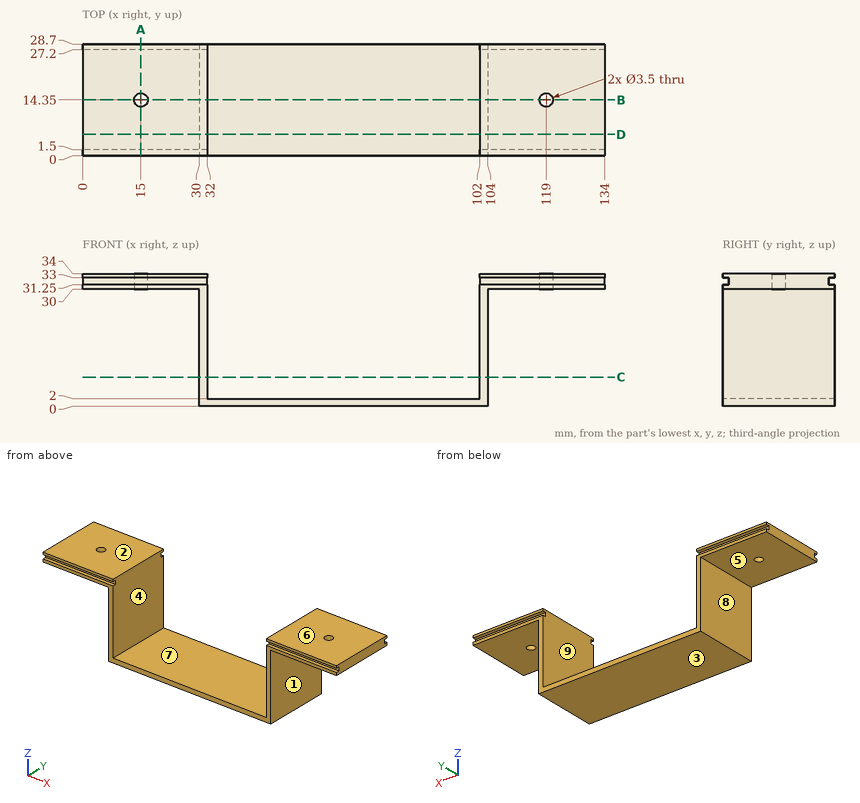
Can you work these out from the drawing? Everything is in mm from the part's minimum corner. A direction names the side the tool comes from. Coordinates: 2 decimals unless noted, no trailing zeros. Loops run counter-clockwise (first coordinate to the right, second up) from the corner with the lowest first, then second, coordinate; pieces in that order, holes last.
1) Which directions (+Z, -Z, +X, -X, +Y, -Y) give clear straight access to the entire face, cutting with the end or side of a thin tool? Please do the marked faces 1, 2, 3, 4 and 5.
2) Imagine slicing it at A-A on x = 15. List the corners of the cut face in (y, z) for me.
3) For pin 1 (1.4 mm diameter, centred on x = 112.5, z = 32, fed in from +Y); pin 2 (1 mm diameter, centred on x = 63, z = 4, fed in from +Y); pin 3 (0.5 mm diameter, centred on x = 115, z = 32.5, fed in from -Y); pin 4 (2 mm diameter, centred on x = 95, y = 13, fed in from +Z), each with a flat end and sliding along its axis, tell me the tip position at first contact or that it passes through.
4) Imagine slicing it at C-C on z = 7.5. List the corners of the cut face in (x, y) for me.
5) Thinking about a two-plate mould opening in X: for the marked faces 6, 7, 8 and 9, which applies, pulls with the +X half, pulls with the -X half, needs draft (parallel to the pull), parting line crosses it, or undercut?
6) I need wall thicknesses on probe 1 along X at (y, z) = (14.35, 32.35); probe 2 along X at (y, z) = (13.5, 30.5); probe 3 along Y at (x, z) = (15, 32.15). Which ranges of each line are inside material? Lowest first, please.
7) Imagine slicing it at D-D on y = 5.5. List the corners of the cut face in (x, z) for me, plus the area to 3 significant figures.
8) Imagine slicing it at B-B on y = 14.35. List the corners of the cut face in (x, z) for me, plus the area to 3 significant figures.
Completed:
1. face 1: -Z, +X, +Y, -Y
1. face 2: +Z, +X, -X, +Y, -Y
1. face 3: -Z, +X, -X, +Y, -Y
1. face 4: +Z, +Y, -Y
1. face 5: -Z, -X, +Y, -Y
2. outline: (0, 30) - (12.6, 30) - (12.6, 34) - (0, 34) - (0, 33) - (1.5, 33) - (1.5, 31.25) - (0, 31.25) - close; (16.1, 30) - (28.7, 30) - (28.7, 31.25) - (27.2, 31.25) - (27.2, 33) - (28.7, 33) - (28.7, 34) - (16.1, 34) - close
3. pin 1: stops at y = 27.2
3. pin 2: passes through
3. pin 3: stops at y = 1.5
3. pin 4: stops at z = 2
4. outline: (30, 0) - (32, 0) - (32, 28.7) - (30, 28.7) - close; (102, 0) - (104, 0) - (104, 28.7) - (102, 28.7) - close
5. face 6: needs draft
5. face 7: undercut
5. face 8: pulls with the -X half
5. face 9: undercut
6. probe 1: x = 0 to 13.25, 16.75 to 32, 102 to 117.25, 120.75 to 134
6. probe 2: x = 0 to 13.47, 16.53 to 32, 102 to 117.47, 120.53 to 134
6. probe 3: y = 1.5 to 12.6, 16.1 to 27.2
7. outline: (0, 30) - (30, 30) - (30, 0) - (104, 0) - (104, 30) - (134, 30) - (134, 34) - (102, 34) - (102, 2) - (32, 2) - (32, 34) - (0, 34) - close
7. area: 516 mm2
8. outline: (0, 30) - (13.25, 30) - (13.25, 34) - (0, 34) - close; (16.75, 30) - (30, 30) - (30, 0) - (104, 0) - (104, 30) - (117.25, 30) - (117.25, 34) - (102, 34) - (102, 2) - (32, 2) - (32, 34) - (16.75, 34) - close; (120.75, 30) - (134, 30) - (134, 34) - (120.75, 34) - close
8. area: 488 mm2
